The drawing under review shows one solid part. Ordinate dimensions are in mm from its lowest x, y, z. A direction names the side the tool comes from. Round coordinates to 2 decimals unless told otherwise and drop trailing zeros. Order: outer loops, then holes, each group sorted by start corner. A loop starts at its lowest first (then second) coordinate and runs counter-clockwise, first axis right, second up. Notation, with made-up numbers: M 82,-22 L 132,-22 A24 cw 132,9 Z; hole C -0.5,21.25 d7. An arc over 180 degrees is marked long. Answer as a JSON object with one key per item and string values.
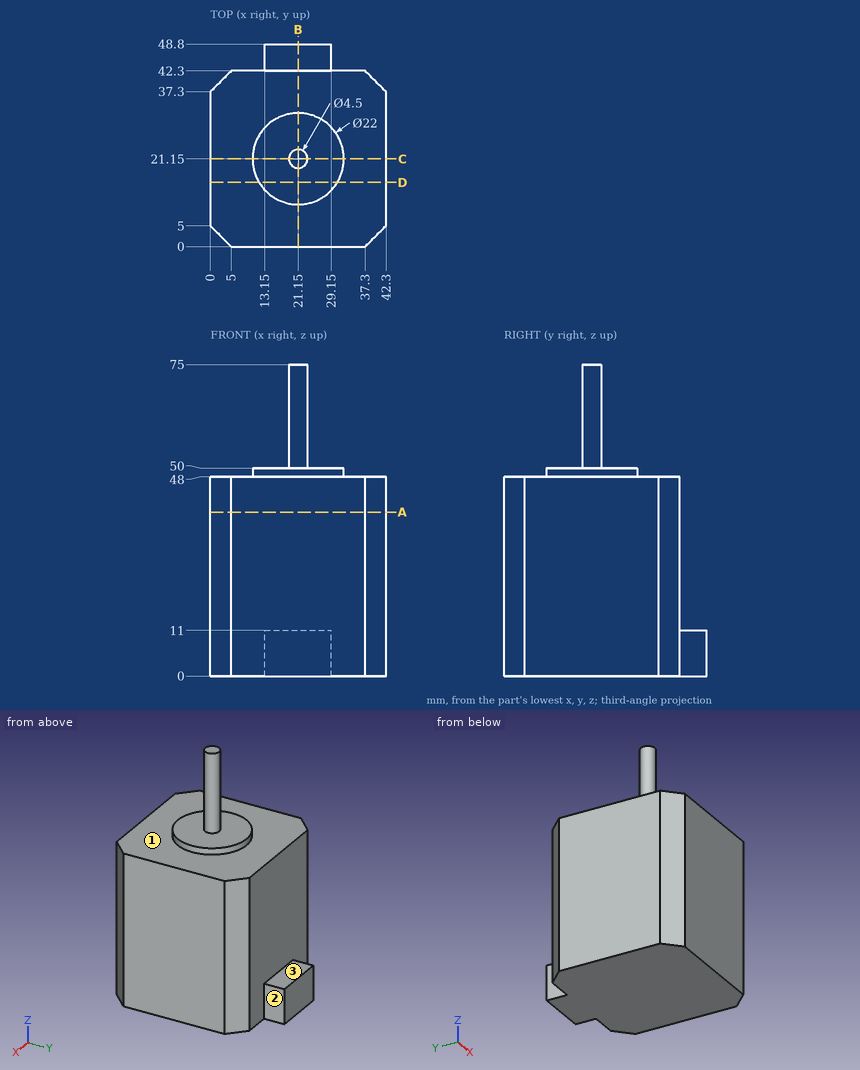
1) Add section A-A on z = 39.5. State the section outline as (x, y) points, and give its area (3 significant figures).
Geometry check:
{"outline": "M 0,5 L 5,0 L 37.3,0 L 42.3,5 L 42.3,37.3 L 37.3,42.3 L 5,42.3 L 0,37.3 Z", "area": "1,740 mm²"}
2) Add section C-C on y = 21.15. State the section outline as (x, z) points, and give its area (3 significant figures).
Geometry check:
{"outline": "M 0,0 L 42.3,0 L 42.3,48 L 32.15,48 L 32.15,50 L 23.4,50 L 23.4,75 L 18.9,75 L 18.9,50 L 10.15,50 L 10.15,48 L 0,48 Z", "area": "2,190 mm²"}
3) Add section B-B on x = 21.15. State the section outline as (y, z) points.
Geometry check:
{"outline": "M 0,0 L 48.8,0 L 48.8,11 L 42.3,11 L 42.3,48 L 32.15,48 L 32.15,50 L 23.4,50 L 23.4,75 L 18.9,75 L 18.9,50 L 10.15,50 L 10.15,48 L 0,48 Z"}
4) Insertion check: P1, Ø5, axis at y = 46, z = 3, coming from the -X side; P2, Ø9.5, axis at x = 26.5, z = 33.5, coming from the +Y side; P3, Ø10, axis at y = 25, z = 66, coming from the -X side. Each pin has a flat end and moves straight along its axis. Give the tip position at first contact, or say it passes through.
Geometry check:
{"P1": "stops at x = 13.15", "P2": "stops at y = 42.3", "P3": "stops at x = 18.9"}
5) Add section D-D on y = 15.5. State the section outline as (x, z) points.
Geometry check:
{"outline": "M 0,0 L 42.3,0 L 42.3,48 L 30.59,48 L 30.59,50 L 11.71,50 L 11.71,48 L 0,48 Z"}
6) Machinability: for the marked faces 1, 2 and 3, which of the approach directions +Z, -Z, +X, -X, +Y, -Y give a long, thin tool a straight path to every point of the face, cutting with its end or side? Answer none if there is none.
Geometry check:
{"face 1": "+Z", "face 2": "+Z, -Z, +X, +Y", "face 3": "+Z, +X, -X, +Y"}
7) For L1, parallel to Z at x = 19, y = 33; L2, parallel to Z at x = 24, y = 22; L3, parallel to Y at x = 9.5, z = 16, list the stretches that pass through material, from the lowest coordinate up.
Geometry check:
{"L1": "z = 0 to 48", "L2": "z = 0 to 50", "L3": "y = 0 to 42.3"}
